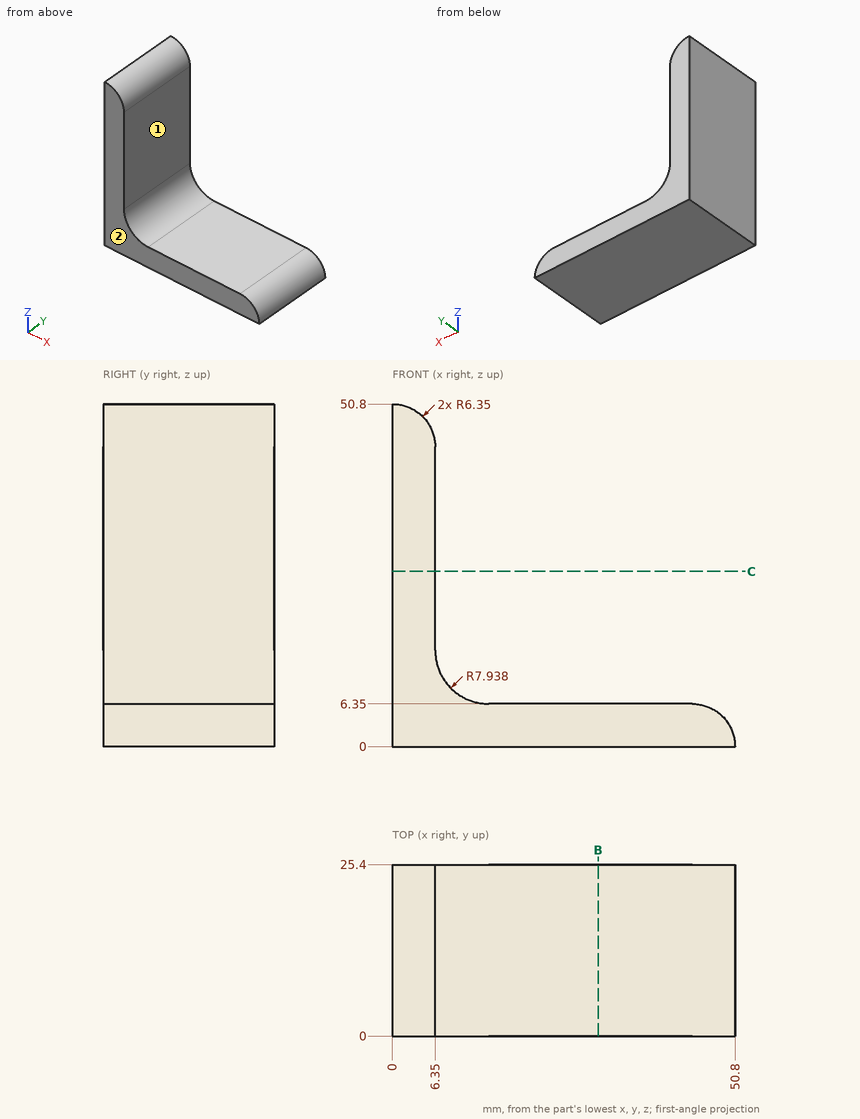
Geometry check sheet. Reference: drawing and pictorial views, mm from the part's lowest x, y, z. A direction names the side the tool comes from. Round coordinates to 2 decimals unless told otherwise and drop trailing zeros. Order: outer loops, then holes, each group sorted by start corner. A loop starts at its lowest first (then second) coordinate and runs counter-clockwise, first axis right, second up. Notation, with made-up numbers: (43.5, -6.5) - (71.5, -6.5) arc R33 ccw to (71.5, 30.5) - close; hole circle Ø2 at (80, -5). An arc over 180 degrees is marked (long way). Use a Markdown table: item, result. Add a question column.
1) Section check B-B (x = 30.5). Record the cut outline in (y, z).
2) Set-up check for the marked faces 1 and 2: record each of +Z, -Z, +X, -X, +Y, -Y from which the full face is reachable in a straight line by a thin tool's end or side.
3) Gauge pin test, flat ends, axial feed: P1, Ø12, axis at y = 9, z = 36, coming from the +X side; P2, Ø4, axis at x = 43.5, y = 4.5, coming from the +Z side; P3, Ø2, axis at x = 6, y = 14, coming from the +Z side (1 decimal). Record the tip position at first contact, or that the pin passes through.
4) Thickness scan on line 1 along Z through (x, y) = (20, 7.5). Record the ranges inside material, lowest first.
5) Section check C-C (z = 26). Record the cut outline in (x, y), then the cut area to 3 significant figures.
Established:
| question | item | result |
|---|---|---|
| 1 | outline | (0, 0) - (25.4, 0) - (25.4, 6.35) - (0, 6.35) - close |
| 2 | face 1 | +Z, +X, +Y, -Y |
| 2 | face 2 | +Z, -Z, +X, -X, -Y |
| 3 | P1 | x = 6.35 |
| 3 | P2 | z = 6.35 |
| 3 | P3 | z = 48.4 |
| 4 | line 1 | 0 to 6.35 |
| 5 | outline | (0, 0) - (6.35, 0) - (6.35, 25.4) - (0, 25.4) - close |
| 5 | area | 161 mm2 |
